Read the model definition and answer for the solid it produces. Units are mm, in the model's axes. Coordinates: 2 decimals unless noted, no trailing zeros. Write each loop counter-clockwise with the first axis right and the second up, starting at its lowest first coordinate (ties: lowest second). Pieces come first, ordered by that corner, then holes. Notation, with made-up numbers: (-5.75, 46.25) - (17.25, 46.25) arc R21 cw to (17.25, 72.25) - close; hole circle Ø11 at (83, 28.5). An arc over 180 degrees is marked (long way). Return JSON: item names as keys, results as strings.
```python
from build123d import *

# Parameters (mm, degrees)
BOSS_EXTRUDE1_DEPTH = 4.191
CUT_EXTRUDE1_START  = -4.191
CUT_EXTRUDE1_DEPTH  = 4.191
CIRPATTERN1_COUNT   = 15
CIRPATTERN1_ANGLE   = 63


with BuildPart() as part:
    # Sketch1 → Boss-Extrude1 (new body)
    with BuildSketch(Plane(origin=(0, 0, 0), x_dir=(1, 0, 0), z_dir=(0, 1, 0))):
        with BuildLine():
            ThreePointArc((-3.275024427, 1.651), (0, 0.762), (3.275024427, 1.651))
            ThreePointArc((3.275024427, 1.651), (3.45634833, -0.274256168), (2.098384379, -1.651))
            ThreePointArc((2.098384379, -1.651), (0, -0.762), (-2.098384379, -1.651))
            ThreePointArc((-2.098384379, -1.651), (-3.45634833, -0.274256168), (-3.275024427, 1.651))
        make_face()
    extrude(amount=BOSS_EXTRUDE1_DEPTH)

    # Sketch2 → Cut-Extrude1 (cut)
    with BuildSketch(Plane(origin=(0, 4.191, 0), x_dir=(1, 0, 0), z_dir=(0, 1, 0)).offset(CUT_EXTRUDE1_START)):
        with BuildLine():
            ThreePointArc((-3.053367923, 1.526866132), (-3.16480485, 1.587846201), (-3.275024427, 1.651))
            Line((-3.275024427, 1.651), (-3.173107841, 1.302860882))
            Line((-3.173107841, 1.302860882), (-3.053367923, 1.526866132))
        make_face()
        with BuildLine():
            Line((-3.053367923, 1.526866132), (-3.173107841, 1.302860882))
            Line((-3.173107841, 1.302860882), (-2.827013928, 1.411520163))
            ThreePointArc((-2.827013928, 1.411520163), (-2.94075651, 1.468083249), (-3.053367923, 1.526866132))
        make_face()
    cut_extrude1 = extrude(amount=CUT_EXTRUDE1_DEPTH, mode=Mode.SUBTRACT)

    # CirPattern1: Cut-Extrude1 ×15 about axis
    cirpattern1_axis = Axis((0, 0, -7.239), (0, 1, 0))
    for i in range(1, CIRPATTERN1_COUNT):
        add(cut_extrude1.rotate(cirpattern1_axis, i * CIRPATTERN1_ANGLE / (CIRPATTERN1_COUNT - 1)), mode=Mode.SUBTRACT)


solid = part.part
```
(1) Flat-ended cylindrical pins translate along their axes: P1, Ø1, axis at y = 0.5, z = 1, coming from the -X side; P2, Ø1, axis at x = -0.5, y = 1, coming from the +Z side. Find the tip coordinate at first contact, or state that the pin passes through.
Answer:
{"P1": "x = -3.36", "P2": "z = 0.94"}
(2) A cutting plane is placed at A-A (z = 1). Determine the outline of the cut face in (x, y).
Answer:
{"outline": "(-3.03, 0) - (-1.15, 0) - (-1.15, 4.19) - (-3.03, 4.19) - close; (1.15, 0) - (3.03, 0) - (3.03, 4.19) - (1.15, 4.19) - close"}
(3) Determine the mould class of faces 1 (the face through (0.033, 2.066, 0.762)), 2 (the face through (0, 0, 0)), 3 (the face through (-3.447, 2.066, 0.301)), 4 (the face through (3.423, 2.066, 0.363)) for opening direction X: +X half, -X half, draft (parallel to the pull), parting line (faces both ways), or undercut.
Answer:
{"face 1": "undercut", "face 2": "draft", "face 3": "-X half", "face 4": "+X half"}
(4) A cutting plane is placed at B-B (x = 1.75). Determine the outline of the cut face in (y, z).
Answer:
{"outline": "(0, -0.91) - (4.19, -0.91) - (4.19, 1.34) - (0, 1.34) - close"}
(5) A cutting plane is placed at C-C (z = 0.35). Determine the outline of the cut face in (x, y).
Answer:
{"outline": "(-3.43, 0) - (3.43, 0) - (3.43, 4.19) - (-3.43, 4.19) - close"}
(6) Straight lines are drawn through the part: line 1 (X direction, y = 1.45, z = 0.55); line 2 (X direction, y = 1.5, z = 1.1); line 3 (Z direction, x = -1, y = 0.5). For each, find the intervals that lie inside material, in ascending order. Write a range as from..to.
Answer:
{"line 1": "-3.34..3.34", "line 2": "-2.94..-1.36, 1.36..2.94", "line 3": "-0.74..0.94"}
